Design review of the part built by this model. Coordinates are the model's own, in mm. Give positions to 0.01 mm unless a question says otherwise; leave off trailing zeros. Loops run counter-clockwise (first coordinate to the right, second up) from the corner with the lowest first, then second, coordinate; pieces in that order, holes last.
from build123d import *

# Parameters (mm, degrees)
MODEL_W                 = 3
MODEL_H                 = 3
SALIENTE_EXTRUIR1_DEPTH = 3


with BuildPart() as part:
    # Model → Saliente-Extruir1 (new body)
    with BuildSketch(Plane.XY):
        with BuildLine():
            Line((9.904781567, 296.774995526), (117.904781567, 296.774995526))
            ThreePointArc((117.904781567, 296.774995526), (122.404781567, 292.274995526), (117.904781567, 287.774995526))
            Line((117.904781567, 287.774995526), (9.904781567, 287.774995526))
            ThreePointArc((9.904781567, 287.774995526), (5.404781567, 292.274995526), (9.904781567, 296.774995526))
        make_face()
        with Locations((9.904781567, 292.274995526)):
            Rectangle(MODEL_W, MODEL_H, mode=Mode.SUBTRACT)
        with Locations((18.904781567, 292.274995526)):
            Rectangle(MODEL_W, MODEL_H, mode=Mode.SUBTRACT)
        with Locations((27.904781567, 292.274995526)):
            Rectangle(MODEL_W, MODEL_H, mode=Mode.SUBTRACT)
        with Locations((36.904781567, 292.274995526)):
            Rectangle(MODEL_W, MODEL_H, mode=Mode.SUBTRACT)
        with Locations((45.904781567, 292.274995526)):
            Rectangle(MODEL_W, MODEL_H, mode=Mode.SUBTRACT)
        with Locations((54.904781567, 292.274995526)):
            Rectangle(MODEL_W, MODEL_H, mode=Mode.SUBTRACT)
        with Locations((63.904781567, 292.274995526)):
            Rectangle(MODEL_W, MODEL_H, mode=Mode.SUBTRACT)
        with Locations((72.904781567, 292.274995526)):
            Rectangle(MODEL_W, MODEL_H, mode=Mode.SUBTRACT)
        with Locations((81.904781567, 292.274995526)):
            Rectangle(MODEL_W, MODEL_H, mode=Mode.SUBTRACT)
        with Locations((90.904781567, 292.274995526)):
            Rectangle(MODEL_W, MODEL_H, mode=Mode.SUBTRACT)
        with Locations((117.904781567, 292.274995526)):
            Rectangle(MODEL_W, MODEL_H, mode=Mode.SUBTRACT)
        with Locations((99.904781567, 292.274995526)):
            Rectangle(MODEL_W, MODEL_H, mode=Mode.SUBTRACT)
        with Locations((108.904781567, 292.274995526)):
            Rectangle(MODEL_W, MODEL_H, mode=Mode.SUBTRACT)
    extrude(amount=SALIENTE_EXTRUIR1_DEPTH)


solid = part.part
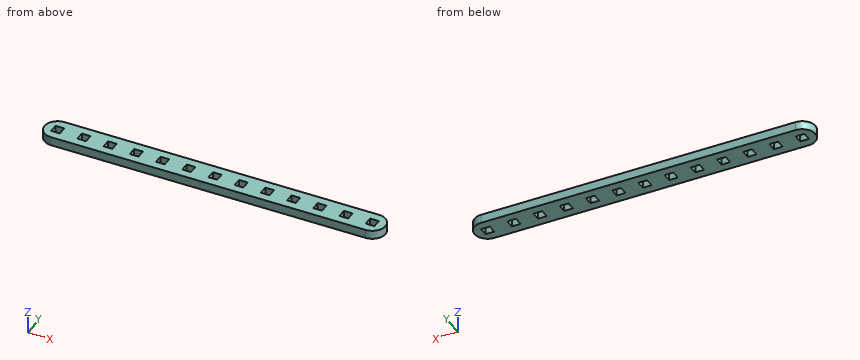
Q1. Take a section at B-B (y = 289.5). Give the boundary of the cut face in (x, z), plus the area to 3 significant figures.
Results:
outline: (6.36, 0) - (121.45, 0) - (121.45, 3) - (6.36, 3) - close
area: 345 mm2
Q2. Take a section at A-A (z = 2.5). Give the number of separate pieces and of enclosed holes in the cut face, plus the area to 3 significant figures.
Results:
separate pieces: 1
enclosed holes: 13
area: 919 mm2
Q3. Wall thickness on line 1 (Y direction, x = 80.5, z = 2.05) (3 decimals); line 2 (X direction, y = 294.75, z = 2.6); line 3 (X direction, y = 295.75, z = 0.8): over which ranges is each line inside the solid? List them lowest first.
Results:
line 1: y = 287.775 to 290.775, 293.775 to 296.775
line 2: x = 6.15 to 121.66
line 3: x = 7.05 to 120.76
